```python
from build123d import *

# Parameters (mm, degrees)
F0_R     = 1.65
F1_DEPTH = 1.6
F2_R     = 4
F3_R     = 6
F4_W     = 2.6
F4_H     = 5.1
F4_H_2   = 1.7
F5_DEPTH = 1.601


with BuildPart() as f1:
    # F0 (on Top) → F1 (new body)
    with BuildSketch(Plane.XY):
        Polygon((0, 35.43), (0, 0), (55.88, 0), (55.88, 22.86), (43.56, 22.86), (43.56, 35.43), (17.27, 35.43), (17.27, 38.35), (4.57, 38.35), (4.57, 35.43), align=None)
        with Locations((3.5, 4.7)):
            Circle(F0_R, mode=Mode.SUBTRACT)
        with Locations((52.58, 4.7)):
            Circle(F0_R, mode=Mode.SUBTRACT)
    extrude(amount=F1_DEPTH)

    # F2
    f2_edges = [f1.edges().sort_by_distance(p)[0] for p in [
        (0, 35.43, 0.8),
    ]]
    fillet(f2_edges, radius=F2_R)

    # F3
    f3_edges = [f1.edges().sort_by_distance(p)[0] for p in [
        (43.56, 22.86, 0.8),
    ]]
    fillet(f3_edges, radius=F3_R)

    # F4 (on face) → F5 (cut, through all)
    with BuildSketch(Plane.XY.offset(1.6)):
        with Locations((11.045, 35.8)):
            Rectangle(F4_W, F4_H)
        with Locations((11.045, 22.3)):
            Rectangle(F4_W, F4_H_2)
    extrude(amount=-F5_DEPTH, mode=Mode.SUBTRACT)


solid = f1.part
```
Source: CAD feature listing. Evaluate the final solid. Frame: model axes, mm. A direction names the side the tool comes from. Round coordinates to 2 decimals unless told otherwise and drop trailing zeros. Order: outer loops, then holes, each group sorted by start corner. A loop starts at its lowest first (then second) coordinate and runs counter-clockwise, first axis right, second up. Notation, with made-up numbers: (65, -11) -> (84, -11) arc R25 cw to (84, 26) -> close; hole circle Ø1 at (24, -3). An arc over 180 degrees is marked (long way). One line per item, written item: value. Start each with the question number.
Q1. Section query D-D (x = 11). Return the cut outline in (y, z).
Q2. Material intervals for probe 1 along X at (y, z) = (4, 1.5); probe 2 along X at (y, z) = (37, 1.45) (3 decimals); probe 3 along X at (y, z) = (22, 0.55) (3 decimals), sorted ascending.
Q3. Section query B-B (y = 4.7). Return the cut outline in (x, z).
Q4. Pin query (flat end, axial travel): pin 1 (0.6 mm diameter, centred on x = 4, z = 0.5, fed in from +Y); pin 2 (0.5 mm diameter, centred on x = 53, z = 0.5, fed in from +Y); pin 3 (0.8 mm diameter, centred on y = 37, z = 1, fed in from +X). Return the tip coordinate at first contact, or that it passes through.
Q5. Section query C-C (x = 52.58). Return the cut outline in (y, z).
Q6. Access query for faces 1 (the flat face through (17.27, 37, 1)), 2 (the flat face through (11, 33.25, 1)), 3 (the flat face through (12.345, 22, 1)), 4 (the flat face through (4.57, 37, 1)). Directions: +Z, -Z, +X, -X, +Y, -Y. A direction counts if a zero-diameter tool reaches every point of the face in a straight line with its end or side. Return the directions, or none.
Q7. Draft query along Y for faces 5 (the flat face through (43.56, 32, 1)), 6 (the flat face through (11, 23.15, 1)), 7 (the flat face through (7, 38.35, 1)). Return one class per face: pulls with the +Y half, pulls with the -Y half, needs draft (parallel to the pull), parting line crosses it, or undercut.
Q8. Section query A-A (z = 0.5). Return the cut outline in (x, y) (3 decimals).
Findings below:
1. outline: (0, 0) -> (21.45, 0) -> (21.45, 1.6) -> (0, 1.6) -> close; (23.15, 0) -> (33.25, 0) -> (33.25, 1.6) -> (23.15, 1.6) -> close
2. probe 1: 0 to 2.01, 4.99 to 51.09, 54.07 to 55.88
2. probe 2: 4.57 to 9.745, 12.345 to 17.27
2. probe 3: 0 to 9.745, 12.345 to 55.88
3. outline: (0, 0) -> (1.85, 0) -> (1.85, 1.6) -> (0, 1.6) -> close; (5.15, 0) -> (50.93, 0) -> (50.93, 1.6) -> (5.15, 1.6) -> close; (54.23, 0) -> (55.88, 0) -> (55.88, 1.6) -> (54.23, 1.6) -> close
4. pin 1: y = 35.43
4. pin 2: y = 22.86
4. pin 3: x = 17.27
5. outline: (0, 0) -> (3.05, 0) -> (3.05, 1.6) -> (0, 1.6) -> close; (6.35, 0) -> (22.86, 0) -> (22.86, 1.6) -> (6.35, 1.6) -> close
6. face 1: +Z, -Z, +X, +Y
6. face 2: +Z, -Z, +Y
6. face 3: +Z, -Z
6. face 4: +Z, -Z, -X, +Y
7. face 5: needs draft
7. face 6: undercut
7. face 7: pulls with the +Y half
8. outline: (0, 0) -> (55.88, 0) -> (55.88, 22.86) -> (49.56, 22.86) arc R6 cw to (43.56, 28.86) -> (43.56, 35.43) -> (17.27, 35.43) -> (17.27, 38.35) -> (12.345, 38.35) -> (12.345, 33.25) -> (9.745, 33.25) -> (9.745, 38.35) -> (4.57, 38.35) -> (4.57, 35.43) -> (4, 35.43) arc R4 ccw to (0, 31.43) -> close; hole circle Ø3.3 at (3.5, 4.7); hole (9.745, 21.45) -> (12.345, 21.45) -> (12.345, 23.15) -> (9.745, 23.15) -> close; hole circle Ø3.3 at (52.58, 4.7)
